Verification items for this drawing (mm, ordinates from the low corner). Round coordinates to 2 decimals unless told otherwise and drop trailing zeros. Order: outer loops, then holes, each group sorted by start corner. A loop starts at its lowest first (then second) coordinate and runs counter-clockwise, first axis right, second up. Notation, with made-up numbers: (-31, -18.5) - (-18, -18.5) arc R23 ccw to (-18, 12.5) - close; hole circle Ø11 at (27, -22.75). An arc over 180 degrees is marked (long way). Return JSON: item names as keys, results as strings. Group by question number.
Q1. Material ranges on line 1 along X through (y, z) = (4.25, 16); line 2 along X through (y, z) = (0.5, 21); line 3 along Y through (x, z) = (29, 13.5), recorded low to high.
Q2. Sectioned sample at D-D, the plane z = 32. Record the cut outline in (x, y).
Q3. Sectioned sample at C-C, the plane x = 8. Record the cut outline in (y, z) (1 decimal).
Q4. Sectioned sample at A-A, the plane z = 12. Record the cut outline in (x, y).
Q5. Draft check along X on the marked faces 1, 2, 3 and 4. Enter one of: pulls with the +X half, pulls with the -X half, needs draft (parallel to the pull), parting line crosses it, or undercut.
Q6. Gauge pin test, flat ends, axial feed: pin 1 Ø3 at (y, z) = (7.5, 25.5) entering from +X; pin 2 Ø2.5 at (y, z) = (4, 15) entering from +X; pin 3 Ø19 at (x, z) = (30, 34.5) entering from +Y; pin 4 Ø1.3 at (x, y) = (9.5, 6.5) entering from +Z (1 decimal). Record the tip position at first contact, or that the pin passes through.
Q7. Sectioned sample at B-B, the plane y = 7.5. Record the cut outline in (x, z) (1 decimal).
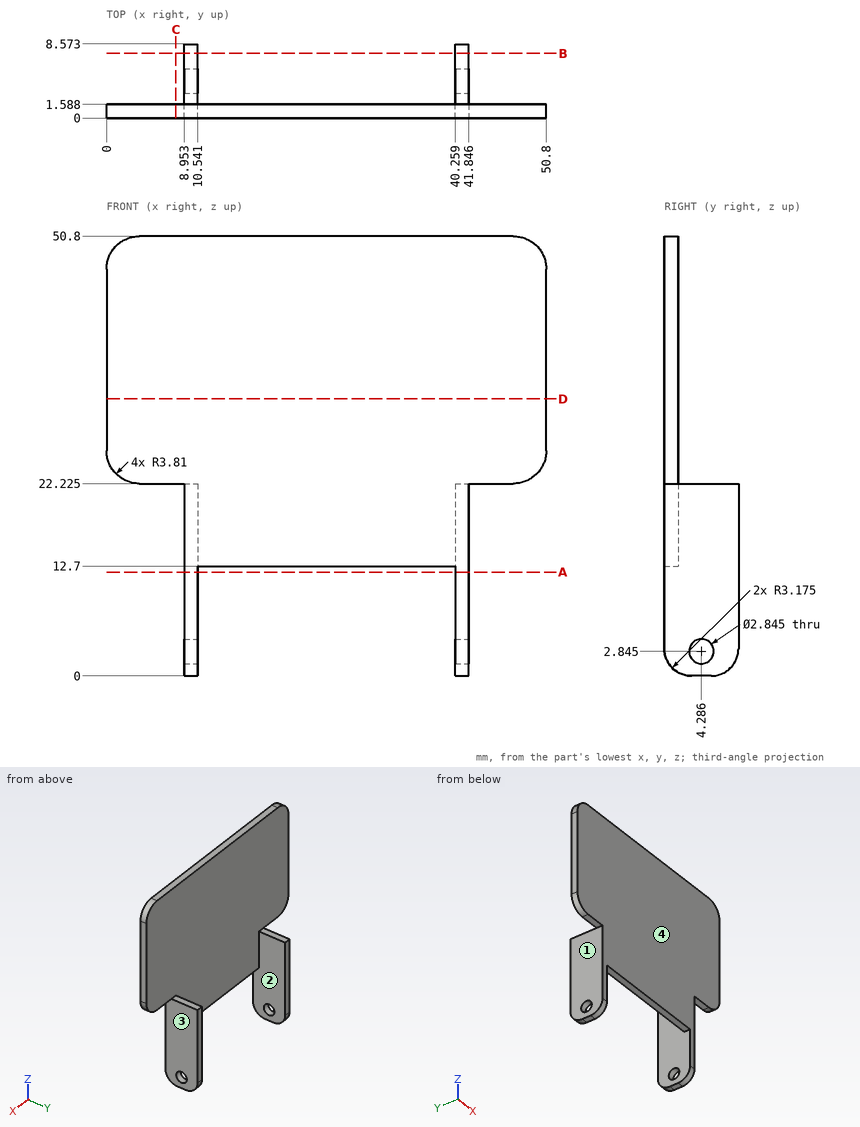
Reply:
{
 "1": {"line 1": "8.95 to 10.54, 40.26 to 41.85", "line 2": "8.95 to 41.85", "line 3": "0 to 1.59"},
 "2": {"outline": "(0, 0) - (50.8, 0) - (50.8, 1.59) - (0, 1.59) - close"},
 "3": {"outline": "(0, 22.2) - (1.6, 22.2) - (1.6, 50.8) - (0, 50.8) - close"},
 "4": {"outline": "(8.95, 0) - (10.54, 0) - (10.54, 8.57) - (8.95, 8.57) - close; (40.26, 0) - (41.85, 0) - (41.85, 8.57) - (40.26, 8.57) - close"},
 "5": {"face 1": "pulls with the -X half", "face 2": "undercut", "face 3": "pulls with the +X half", "face 4": "needs draft"},
 "6": {"pin 1": "through", "pin 2": "x = 41.85", "pin 3": "y = 1.59", "pin 4": "z = 22.2"},
 "7": {"outline": "(9, 0.8) - (10.5, 0.8) - (10.5, 22.2) - (9, 22.2) - close; (40.3, 0.8) - (41.8, 0.8) - (41.8, 22.2) - (40.3, 22.2) - close"}
}
